Design review of the part built by this model. Coordinates are the model's own, in mm. A direction names the side the tool comes from. Give positions to 0.01 mm unless a question says otherwise; leave off trailing zeros. Order: outer loops, then holes, each group sorted by start corner. A loop starts at its lowest first (then second) coordinate and runs counter-clockwise, first axis right, second up. Notation, with made-up numbers: M 65.25,39.25 L 82.25,39.25 A16 cw 82.25,52.25 Z; hole C 26,14 d7. An arc over 180 degrees is marked long. Put each result on its own line as item: value. Start each with the question number.
from build123d import *

# Parameters (mm, degrees)
SKETCH1_W           = 101.6
SKETCH1_H           = 17.78
SKETCH1_R           = 3.96875
BOSS_EXTRUDE1_DEPTH = 33.02
SKETCH2_R           = 2.4892
CUT_EXTRUDE1_DEPTH  = 17.78
SKETCH3_R           = 4.064
CUT_EXTRUDE2_DEPTH  = 4.826
CUT_EXTRUDE3_DEPTH  = 109.300548475
FILLET1_R           = 2.54
CUT_EXTRUDE4_DEPTH  = 106.921350067


with BuildPart() as part:
    # Sketch1 → Boss-Extrude1 (new body)
    with BuildSketch(Plane(origin=(0, 0, 0), x_dir=(1, 0, 0), z_dir=(0, 1, 0))):
        with Locations((50.8, 8.89)):
            Rectangle(SKETCH1_W, SKETCH1_H)
        with Locations(Location((76.2, 8.89, 0), (0, 0, 270))):
            Circle(SKETCH1_R, mode=Mode.SUBTRACT)
        with Locations(Location((25.4, 8.89, 0), (0, 0, 270))):
            Circle(SKETCH1_R, mode=Mode.SUBTRACT)
    extrude(amount=-BOSS_EXTRUDE1_DEPTH)

    # Sketch2 → Cut-Extrude1 (cut)
    with BuildSketch(Plane.XY):
        with Locations((88.9, -16.51)):
            Circle(SKETCH2_R)
        with Locations((12.7, -16.51)):
            Circle(SKETCH2_R)
    extrude(amount=-CUT_EXTRUDE1_DEPTH, mode=Mode.SUBTRACT)

    # Sketch3 → Cut-Extrude2 (cut)
    with BuildSketch(Plane.XY):
        with Locations((88.9, -16.51)):
            Circle(SKETCH3_R)
        with Locations((12.7, -16.51)):
            Circle(SKETCH3_R)
    extrude(amount=-CUT_EXTRUDE2_DEPTH, mode=Mode.SUBTRACT)

    # Sketch5 → Cut-Extrude3 (cut, through all)
    with BuildSketch(Plane.XY):
        with BuildLine():
            Line((12.7, -5.150774674), (12.7, 0))
            Line((12.7, 0), (0, 0))
            Line((0, 0), (0, -33.02))
            Line((0, -33.02), (12.7, -33.02))
            Line((12.7, -33.02), (12.7, -27.869225326))
            ThreePointArc((12.7, -27.869225326), (12.37660211, -27.022558659), (11.571111111, -26.607089178))
            ThreePointArc((11.571111111, -26.607089178), (2.54, -16.51), (11.571111111, -6.412910822))
            ThreePointArc((11.571111111, -6.412910822), (12.37660211, -5.997441341), (12.7, -5.150774674))
        make_face()
        with BuildLine():
            Line((88.9, -5.150774674), (88.9, 0))
            Line((88.9, 0), (101.6, 0))
            Line((101.6, 0), (101.6, -33.02))
            Line((101.6, -33.02), (88.9, -33.02))
            Line((88.9, -33.02), (88.9, -27.869225326))
            ThreePointArc((88.9, -27.869225326), (89.22339789, -27.022558659), (90.028888889, -26.607089178))
            ThreePointArc((90.028888889, -26.607089178), (99.06, -16.51), (90.028888889, -6.412910822))
            ThreePointArc((90.028888889, -6.412910822), (89.22339789, -5.997441341), (88.9, -5.150774674))
        make_face()
    extrude(amount=-CUT_EXTRUDE3_DEPTH, mode=Mode.SUBTRACT)

    # Fillet1
    fillet1_edges = [part.edges().sort_by_distance(p)[0] for p in [
        (12.7, -33.02, -8.89),
        (12.7, 0, -8.89),
        (88.9, 0, -8.89),
        (88.9, -33.02, -8.89),
    ]]
    fillet(fillet1_edges, radius=FILLET1_R)

    # Sketch6 → Cut-Extrude4 (cut, through all)
    with BuildSketch(Plane.XY):
        with BuildLine():
            Line((38.1, -27.94), (63.5, -27.94))
            ThreePointArc((63.5, -27.94), (65.296051224, -27.196051224), (66.04, -25.4))
            Line((66.04, -25.4), (66.04, -7.62))
            ThreePointArc((66.04, -7.62), (65.296051224, -5.823948776), (63.5, -5.08))
            Line((63.5, -5.08), (38.1, -5.08))
            ThreePointArc((38.1, -5.08), (36.303948776, -5.823948776), (35.56, -7.62))
            Line((35.56, -7.62), (35.56, -25.4))
            ThreePointArc((35.56, -25.4), (36.303948776, -27.196051224), (38.1, -27.94))
        make_face()
    extrude(amount=-CUT_EXTRUDE4_DEPTH, mode=Mode.SUBTRACT)


solid = part.part
1. Consider section A-A on y = -16.51. Give the boundary of the cut face in (x, z).
2. Consider section B-B on z = -8.89. Give the number of separate pieces and of enclosed holes in the cut face, then the cut area to 3 significant figures.
3. Consider section C-C on x = 76.2. Give the boundary of the cut face in (y, z), then the cut area to 3 significant figures.
4. Machinability: for faces 1 (the cylindrical face through (36.284, -27.176, -8.766)), 2 (the flat face through (12.7, -29, -9)), 3 (the cylindrical face through (85.905, -13.763, -2.379)), which of the approach directions +Z, -Z, +X, -X, +Y, -Y give a long, thin tool a straight path to every point of the face, cutting with its end or side? Answer none if there is none.
5. Consider section D-D on y = -22.5. Give the boundary of the cut face in (x, z).
6. Insertion check: pin 1 (1.5 mm diameter, centred on y = -8, z = -11, fed in from +X); pin 2 (0.8 mm diameter, centred on y = -3.5, z = -5, fed in from -X); pin 3 (4.5 mm diameter, centred on x = 12.7, y = -16.51, fed in from -Z); pin 4 (7.5 mm diameter, centred on x = 88.9, y = -16.51, fed in from +Z). Each pin has a flat end and moves straight along its axis. Give the tip position at first contact, or say it passes through.
7. The part is to be moulded in two halves that separate along Z. For faces 4 (the cylindrical face through (79.55, -16.28, -6.76)), 5 (the flat face through (12.6, -19.2, -4.826)), 6 (the flat face through (51, -27.94, -9)), say which applies: +Z half, -Z half, draft (parallel to the pull), parting line (faces both ways), or undercut.
8. To check wall thickness, follow probe 1 along Y at (x, z) = (37.5, -7.25); probe 2 along X at (y, z) = (-8, -9); probe 3 along X at (y, z) = (-4.5, -8.75). State the ranges of each line that lie inside material, in increasing order.
Returned:
1. outline: M 2.54,-17.78 L 10.21,-17.78 L 10.21,-4.83 L 8.64,-4.83 L 8.64,0 L 2.54,0 Z; M 15.19,-17.78 L 35.56,-17.78 L 35.56,0 L 16.76,0 L 16.76,-4.83 L 15.19,-4.83 Z; M 66.04,-17.78 L 86.41,-17.78 L 86.41,-4.83 L 84.84,-4.83 L 84.84,0 L 66.04,0 Z; M 91.39,-17.78 L 99.06,-17.78 L 99.06,0 L 92.96,0 L 92.96,-4.83 L 91.39,-4.83 Z; hole C 25.4,-8.89 d7.94; hole C 76.2,-8.89 d7.94
2. separate pieces: 3
2. enclosed holes: 3
2. area: 1,580 mm2
3. outline: M -33.02,-17.78 L 0,-17.78 L 0,-12.86 L -33.02,-12.86 Z; M -33.02,-4.92 L 0,-4.92 L 0,0 L -33.02,0 Z
3. area: 325 mm2
4. face 1: +Z, -Z
4. face 2: +Z, -Z, -X, -Y
4. face 3: +Z
5. outline: M 4.49,-17.78 L 35.56,-17.78 L 35.56,0 L 4.49,0 Z; M 66.04,-17.78 L 97.11,-17.78 L 97.11,0 L 66.04,0 Z; hole C 25.4,-8.89 d7.94; hole C 76.2,-8.89 d7.94
6. pin 1: stops at x = 95.46
6. pin 2: stops at x = 12.7
6. pin 3: passes through
6. pin 4: stops at z = -4.83
7. face 4: undercut
7. face 5: +Z half
7. face 6: draft
8. probe 1: y = -33.02 to -27.87, -5.15 to 0
8. probe 2: x = 7.15 to 21.43, 29.37 to 35.56, 66.04 to 72.23, 80.17 to 94.45
8. probe 3: x = 12.7 to 21.43, 29.37 to 72.23, 80.17 to 88.9
